```python
from build123d import *

# Parameters (mm, degrees)
SKETCH1_R                   = 6.35
HANDLE_BASE_DEPTH           = 38.1
F_1_4_20_TAPPED_HOLE1_D     = 5.1054
F_1_4_20_TAPPED_HOLE1_DEPTH = 22.596183098
F_1_4_20_TAPPED_HOLE1_TIP   = 1.533816902
SKETCH2_R                   = 2.5527
CUT_EXTRUDE1_DEPTH          = 40.144028919


with BuildPart() as part:
    # Sketch1 → Handle Base (new body)
    with BuildSketch(Plane.XY):
        with Locations(Location((0, 0, 0), (0, 0, 180))):
            Circle(SKETCH1_R)
    extrude(amount=HANDLE_BASE_DEPTH)

    # 1/4-20 Tapped Hole1
    with Locations(Plane.XY.offset(38.1)):
        with Locations((0, 0)):
            Hole(F_1_4_20_TAPPED_HOLE1_D / 2, depth=F_1_4_20_TAPPED_HOLE1_DEPTH)
            with Locations((0, 0, -(F_1_4_20_TAPPED_HOLE1_DEPTH + F_1_4_20_TAPPED_HOLE1_TIP / 2))):  # 118° drill point
                Cone(0, F_1_4_20_TAPPED_HOLE1_D / 2, F_1_4_20_TAPPED_HOLE1_TIP, mode=Mode.SUBTRACT)

    # Sketch2 → Cut-Extrude1 (cut, through all)
    with BuildSketch(Plane.XY.offset(38.1)):
        Circle(SKETCH2_R)
    extrude(amount=-CUT_EXTRUDE1_DEPTH, mode=Mode.SUBTRACT)


solid = part.part
```
Check sheet for the modelled part. Datum: model origin and axes. Units: mm. Coordinates: 2 decimals unless noted, no trailing zeros. Loops run counter-clockwise (first coordinate to the right, second up) from the corner with the lowest first, then second, coordinate; pieces in that order, holes last.
1) Material ranges on probe 1 along Y at (x, z) = (0, 8); probe 2 along Y at (x, z) = (-1.5, 32); probe 3 along X at (y, z) = (2.25, 8), recorded low to high.
2) Sectioned sample at B-B (y = -1). Record the boundary of the cut face in (x, z), and give its area (3 significant figures).
3) Sectioned sample at D-D (y = 3.25). Record the boundary of the cut face in (x, z), and give its area (3 significant figures).
4) Sectioned sample at C-C (z = 23.5). Record the boundary of the cut face in (x, y).
5) Sectioned sample at A-A (x = 0). Record the boundary of the cut face in (y, z), and give its area (3 significant figures).
6) Gauge pin test, flat ends, axial feed: pin 1 (4 mm diameter, centred on y = 3.5, z = 4, fed in from +X); pin 2 (4 mm diameter, centred on x = 0, y = 0, fed in from +Z); pin 3 (6 mm diameter, centred on x = 3.5, z = 10.5, fed in from +Y); pin 4 (4 mm diameter, centred on x = 3.5, z = 11.5, fed in from -Y). Record the tip position at first contact, or that the pin passes through.
Check sheet entries:
1. probe 1: y = -6.35 to -2.55, 2.55 to 6.35
1. probe 2: y = -6.17 to -2.07, 2.07 to 6.17
1. probe 3: x = -5.94 to -1.21, 1.21 to 5.94
2. outline: (-6.27, 0) - (-2.35, 0) - (-2.35, 38.1) - (-6.27, 38.1) - close; (2.35, 0) - (6.27, 0) - (6.27, 38.1) - (2.35, 38.1) - close
2. area: 299 mm2
3. outline: (-5.46, 0) - (5.46, 0) - (5.46, 38.1) - (-5.46, 38.1) - close
3. area: 416 mm2
4. outline: circle Ø12.7 at (0, 0); hole circle Ø5.11 at (0, 0)
5. outline: (-6.35, 0) - (-2.55, 0) - (-2.55, 38.1) - (-6.35, 38.1) - close; (2.55, 0) - (6.35, 0) - (6.35, 38.1) - (2.55, 38.1) - close
5. area: 289 mm2
6. pin 1: stops at x = 6.17
6. pin 2: passes through
6. pin 3: stops at y = 6.33
6. pin 4: stops at y = -6.17
